Verification items for the finished model (mm, model axes). A direction names the side the tool comes from. Coordinates: 2 decimals unless noted, no trailing zeros. Write each loop counter-clockwise with the first axis right and the second up, starting at its lowest first coordinate (ties: lowest second). Pieces come first, ordered by that corner, then holes. Notation, with made-up numbers: M -12.75,25.5 L 4.25,25.5 A29 cw 4.25,56.5 Z; hole C 40.25,65.25 d6. An arc over 180 degrees is marked long. One line per item, written item: value.
```python
from build123d import *

# Parameters (mm, degrees)
BOSS_EXTRUDE1_DEPTH     = 5
CUT_EXTRUDE1_DEPTH      = 11.43956726
CUT_EXTRUDE1_DEPTH_BACK = 11.43956726
SKETCH2_R               = 2.65


with BuildPart() as part:
    # Sketch1 → Boss-Extrude1 (new body)
    with BuildSketch(Plane.XZ.offset(5)):
        with BuildLine():
            Line((3.190229537, -2.808012732), (3.879551376, -3.414747915))
            add(Edge.make_bspline(
                [(3.879551376, -3.414747915), (4.371081204, -3.768547035), (5.325327031, -3.7270487)],
                knots=[3.664389894, 3.664389894, 3.664389894, 4.719659584, 4.719659584, 4.719659584], degree=2, weights=[1, 0.864000321, 1]))
            Line((5.325327031, -3.7270487), (5.602463544, -3.295815869))
            add(Edge.make_bspline(
                [(5.602463544, -3.295815869), (5.243842932, -2.409552511), (4.717787845, -2.11042651)],
                knots=[1.542822379, 1.542822379, 1.542822379, 2.616695251, 2.616695251, 2.616695251], degree=2, weights=[1, 0.859279742, 1]))
            Line((4.717787845, -2.11042651), (3.879527469, -1.735444214))
            ThreePointArc((3.879527469, -1.735444214), (4.077845138, -1.197363367), (4.201918167, -0.637482326))
            Line((4.201918167, -0.637482326), (5.109838405, -0.775224919))
            add(Edge.make_bspline(
                [(5.109838405, -0.775224919), (5.714617855, -0.807118591), (6.494944834, -0.256303727)],
                knots=[3.664389894, 3.664389894, 3.664389894, 4.719659584, 4.719659584, 4.719659584], degree=2, weights=[1, 0.864000321, 1]))
            Line((6.494944834, -0.256303727), (6.494944834, 0.256303727))
            add(Edge.make_bspline(
                [(6.494944834, 0.256303727), (5.714103832, 0.807990967), (5.109838405, 0.775224919)],
                knots=[1.542822379, 1.542822379, 1.542822379, 2.616695251, 2.616695251, 2.616695251], degree=2, weights=[1, 0.859279742, 1]))
            Line((5.109838405, 0.775224919), (4.201918167, 0.637482326))
            ThreePointArc((4.201918167, 0.637482326), (4.077845138, 1.197363367), (3.879527469, 1.735444214))
            Line((3.879527469, 1.735444214), (4.717787845, 2.11042651))
            add(Edge.make_bspline(
                [(4.717787845, 2.11042651), (5.243803714, 2.410564302), (5.602463544, 3.295815869)],
                knots=[0.52279724, 0.52279724, 0.52279724, 1.57806693, 1.57806693, 1.57806693], degree=2, weights=[1, 0.864000321, 1]))
            Line((5.602463544, 3.295815869), (5.325327031, 3.7270487))
            add(Edge.make_bspline(
                [(5.325327031, 3.7270487), (4.370177139, 3.769003022), (3.879551376, 3.414747915)],
                knots=[1.542822379, 1.542822379, 1.542822379, 2.616695251, 2.616695251, 2.616695251], degree=2, weights=[1, 0.859279742, 1]))
            Line((3.879551376, 3.414747915), (3.190229537, 2.808012732))
            ThreePointArc((3.190229537, 2.808012732), (2.783158119, 3.211935691), (2.32541421, 3.557379478))
            Line((2.32541421, 3.557379478), (2.827872978, 4.326032434))
            add(Edge.make_bspline(
                [(2.827872978, 4.326032434), (3.108118945, 4.862910062), (2.931239663, 5.801537213)],
                knots=[0.52279724, 0.52279724, 0.52279724, 1.57806693, 1.57806693, 1.57806693], degree=2, weights=[1, 0.864000321, 1]))
            Line((2.931239663, 5.801537213), (2.464955522, 6.014482045))
            add(Edge.make_bspline(
                [(2.464955522, 6.014482045), (1.638750082, 5.533383248), (1.417534197, 4.970112574)],
                knots=[1.542822379, 1.542822379, 1.542822379, 2.616695251, 2.616695251, 2.616695251], degree=2, weights=[1, 0.859279742, 1]))
            Line((1.417534197, 4.970112574), (1.16566557, 4.087018936))
            ThreePointArc((1.16566557, 4.087018936), (0.604838063, 4.206741128), (0.032998371, 4.249871893))
            Line((0.032998371, 4.249871893), (0.040128421, 5.168153627))
            add(Edge.make_bspline(
                [(0.040128421, 5.168153627), (-0.014371628, 5.771316237), (-0.670632099, 6.465311484)],
                knots=[0.52279724, 0.52279724, 0.52279724, 1.57806693, 1.57806693, 1.57806693], degree=2, weights=[1, 0.864000321, 1]))
            Line((-0.670632099, 6.465311484), (-1.178021948, 6.392359837))
            add(Edge.make_bspline(
                [(-1.178021948, 6.392359837), (-1.612968547, 5.54095339), (-1.494540074, 4.947501609)],
                knots=[4.684415032, 4.684415032, 4.684415032, 5.758287905, 5.758287905, 5.758287905], degree=2, weights=[1, 0.859279742, 1]))
            Line((-1.494540074, 4.947501609), (-1.22898898, 4.068425505))
            ThreePointArc((-1.22898898, 4.068425505), (-1.765513805, 3.86593598), (-2.269894218, 3.59306001))
            Line((-2.269894218, 3.59306001), (-2.760356625, 4.369422559))
            add(Edge.make_bspline(
                [(-2.760356625, 4.369422559), (-3.132299311, 4.847370285), (-4.059582909, 5.076395041)],
                knots=[0.52279724, 0.52279724, 0.52279724, 1.57806693, 1.57806693, 1.57806693], degree=2, weights=[1, 0.864000321, 1]))
            Line((-4.059582909, 5.076395041), (-4.446985774, 4.740708547))
            add(Edge.make_bspline(
                [(-4.446985774, 4.740708547), (-4.352581058, 3.789309981), (-3.932108431, 3.35409384)],
                knots=[4.684415032, 4.684415032, 4.684415032, 5.758287905, 5.758287905, 5.758287905], degree=2, weights=[1, 0.859279742, 1]))
            Line((-3.932108431, 3.35409384), (-3.233448212, 2.758135722))
            ThreePointArc((-3.233448212, 2.758135722), (-3.575327515, 2.297723474), (-3.852111431, 1.795476962))
            Line((-3.852111431, 1.795476962), (-4.684447947, 2.183430702))
            add(Edge.make_bspline(
                [(-4.684447947, 2.183430702), (-5.255744094, 2.384418517), (-6.159644828, 2.07575904)],
                knots=[0.52279724, 0.52279724, 0.52279724, 1.57806693, 1.57806693, 1.57806693], degree=2, weights=[1, 0.864000321, 1]))
            Line((-6.159644828, 2.07575904), (-6.304063037, 1.58391579))
            add(Edge.make_bspline(
                [(-6.304063037, 1.58391579), (-5.710279838, 0.834587427), (-5.121260145, 0.695784976)],
                knots=[4.684415032, 4.684415032, 4.684415032, 5.758287905, 5.758287905, 5.758287905], degree=2, weights=[1, 0.859279742, 1]))
            Line((-5.121260145, 0.695784976), (-4.211310483, 0.572157336))
            ThreePointArc((-4.211310483, 0.572157336), (-4.25, 0), (-4.211310483, -0.572157336))
            Line((-4.211310483, -0.572157336), (-5.121260145, -0.695784976))
            add(Edge.make_bspline(
                [(-5.121260145, -0.695784976), (-5.710527263, -0.835569283), (-6.304063037, -1.58391579)],
                knots=[3.664389894, 3.664389894, 3.664389894, 4.719659584, 4.719659584, 4.719659584], degree=2, weights=[1, 0.864000321, 1]))
            Line((-6.304063037, -1.58391579), (-6.159644828, -2.07575904))
            add(Edge.make_bspline(
                [(-6.159644828, -2.07575904), (-5.255005116, -2.385110738), (-4.684447947, -2.183430702)],
                knots=[4.684415032, 4.684415032, 4.684415032, 5.758287905, 5.758287905, 5.758287905], degree=2, weights=[1, 0.859279742, 1]))
            Line((-4.684447947, -2.183430702), (-3.852111431, -1.795476962))
            ThreePointArc((-3.852111431, -1.795476962), (-3.575327515, -2.297723474), (-3.233448212, -2.758135722))
            Line((-3.233448212, -2.758135722), (-3.932108431, -3.35409384))
            add(Edge.make_bspline(
                [(-3.932108431, -3.35409384), (-4.352258375, -3.790269739), (-4.446985774, -4.740708547)],
                knots=[3.664389894, 3.664389894, 3.664389894, 4.719659584, 4.719659584, 4.719659584], degree=2, weights=[1, 0.864000321, 1]))
            Line((-4.446985774, -4.740708547), (-4.059582909, -5.076395041))
            add(Edge.make_bspline(
                [(-4.059582909, -5.076395041), (-3.1313034, -4.847553096), (-2.760356625, -4.369422559)],
                knots=[4.684415032, 4.684415032, 4.684415032, 5.758287905, 5.758287905, 5.758287905], degree=2, weights=[1, 0.859279742, 1]))
            Line((-2.760356625, -4.369422559), (-2.269894218, -3.59306001))
            ThreePointArc((-2.269894218, -3.59306001), (-1.765513805, -3.86593598), (-1.22898898, -4.068425505))
            Line((-1.22898898, -4.068425505), (-1.494540074, -4.947501609))
            add(Edge.make_bspline(
                [(-1.494540074, -4.947501609), (-1.612178204, -5.541586333), (-1.178021948, -6.392359837)],
                knots=[3.664389894, 3.664389894, 3.664389894, 4.719659584, 4.719659584, 4.719659584], degree=2, weights=[1, 0.864000321, 1]))
            Line((-1.178021948, -6.392359837), (-0.670632099, -6.465311484))
            add(Edge.make_bspline(
                [(-0.670632099, -6.465311484), (-0.013434979, -5.770931598), (0.040128421, -5.168153627)],
                knots=[1.542822379, 1.542822379, 1.542822379, 2.616695251, 2.616695251, 2.616695251], degree=2, weights=[1, 0.859279742, 1]))
            Line((0.040128421, -5.168153627), (0.032998371, -4.249871893))
            ThreePointArc((0.032998371, -4.249871893), (0.604838063, -4.206741128), (1.16566557, -4.087018936))
            Line((1.16566557, -4.087018936), (1.417534197, -4.970112574))
            add(Edge.make_bspline(
                [(1.417534197, -4.970112574), (1.639757156, -5.533488422), (2.464955522, -6.014482045)],
                knots=[3.664389894, 3.664389894, 3.664389894, 4.719659584, 4.719659584, 4.719659584], degree=2, weights=[1, 0.864000321, 1]))
            Line((2.464955522, -6.014482045), (2.931239663, -5.801537213))
            add(Edge.make_bspline(
                [(2.931239663, -5.801537213), (3.108698953, -4.862080092), (2.827872978, -4.326032434)],
                knots=[1.542822379, 1.542822379, 1.542822379, 2.616695251, 2.616695251, 2.616695251], degree=2, weights=[1, 0.859279742, 1]))
            Line((2.827872978, -4.326032434), (2.32541421, -3.557379478))
            ThreePointArc((2.32541421, -3.557379478), (2.783158119, -3.211935691), (3.190229537, -2.808012732))
        make_face()
    extrude(amount=-BOSS_EXTRUDE1_DEPTH)

    # Sketch2 → Cut-Extrude1 (cut, two sides: drawn at the far end of the back side and taken through both)
    with BuildSketch(Plane(origin=(0, 0, 0), x_dir=(1, 0, 0), z_dir=(0, 1, 0)).offset(-CUT_EXTRUDE1_DEPTH_BACK)):
        with Locations(Location((0, 0, 0), (0, 0, 270))):
            Circle(SKETCH2_R)
    extrude(amount=CUT_EXTRUDE1_DEPTH + CUT_EXTRUDE1_DEPTH_BACK, mode=Mode.SUBTRACT)


solid = part.part
```
Item 1: Go/stop test with flat-tipped pins: P1, Ø1.5, axis at x = -4, y = -1.5, coming from the -Z side; P2, Ø3, axis at x = -0.5, z = -2.5, coming from the +Y side. Record where each tip stops, or that it passes through.
The answers:
P1: stops at z = -5.08
P2: stops at y = 0
Item 2: Draft check along Z on faces 1 (the face through (1.29, -2.54, -4.52)), 2 (the face through (-1.364, -2.535, 4.514)), 3 (the face through (-3, 0, 0)). Enter one of: released by +Z, released by -Z, zero draft, split by the parting line, or undercut.
The answers:
face 1: released by -Z
face 2: undercut
face 3: zero draft
Item 3: Scan lines: line 1 (X direction, y = -3.6, z = 0); line 2 (Z direction, x = 5.5, y = -2.55); line 3 (Z direction, x = -5, y = -4.2). Record each from-to range of solid material in increasing order.
The answers:
line 1: x = -4.25 to -2.65, 2.65 to 6.49
line 2: z = -3.46 to -3.07, -0.73 to 0.73, 3.07 to 3.46
line 3: z = -2.25 to -0.68, 0.68 to 2.25
Item 4: Cross-section at A-A, the plane z = 0. Enter the section's corners in (x, y).
The answers:
outline: M -4.25,-5 L -2.65,-5 L -2.65,0 L -4.25,0 Z; M 2.65,-5 L 6.49,-5 L 6.49,0 L 2.65,0 Z
Item 5: Access from +Z, -Z, +X, -X, +Y, -Y to the whole of each face (thin tool, end or side, straight path). Record for faces 4 (the face through (4.662, -2.535, 0.707)), 5 (the face through (4.29, -2.54, 1.92)), 6 (the face through (-3, -5, 0)), 7 (the face through (-4.66, -2.535, -0.633)).
The answers:
face 4: +Y, -Y
face 5: +X, +Y, -Y
face 6: +Z, -Z, +X, -X, -Y
face 7: -X, +Y, -Y
